Autodesk Inventor part; units mm, degrees
ref_plane "YZ Plane" through (0, 0, 0) normal (1, 0, 0) x (0, 1, 0)
ref_plane "XZ Plane" through (0, 0, 0) normal (0, 1, 0) x (-1, 0, 0)
ref_plane "XY Plane" through (0, 0, 0) normal (0, 0, 1) x (1, 0, 0)
sketch "Sketch1" plane through (0, 0, 0) normal (0, 1, 0) x (-1, 0, 0)
  line L0 (5, 5) -> (-5, 5)
  line L1 (-5, 5) -> (-5, -5)
  line L2 (-5, -5) -> (5, -5)
  line L3 (5, -5) -> (5, 5)
  point P0 (0, 0)
  dimension "d0" = 10
  dimension "d1" = 10
extrude "Extrusion1" add sketch "Sketch1" along normal blind 10
sketch "Sketch2" plane through (5, 0, 5) normal (1, 0, 0) x (0, 0, -1)
  line L0 (0, 0) -> (10, 0) construction
  line L1 (10, 0) -> (10, 10) construction
  line L2 (0, 10) -> (10, 10) construction
  line L3 (0, 0) -> (0, 10) construction
  line L4 (0, 10) -> (10, 10) construction
  line L5 (5, 10) -> (5, 0) construction
  line L6 (0, 0) -> (0, 10) construction
  line L7 (0, 5) -> (10, 5) construction
  line L8 (10, 0) -> (10, 10) construction
  circle A0 centre (5, 5) radius 2.5
  dimension "d4" = 5
extrude "Extrusion2" cut sketch "Sketch2" against normal blind 2
properties part number "cubo_calibracion_1cm"
Geometry check sheet. Reference: the model listing, model coordinates, mm. A direction names the side the tool comes from. Give positions to 0.01 mm unless a question says otherwise; leave off trailing zeros. Write each loop counter-clockwise with the first axis right and the second up, starting at its lowest first coordinate (ties: lowest second). Pieces come first, ordered by that corner, then holes. Notation, with made-up numbers: M -39.75,-30.5 L 8.25,-30.5 A22 ccw 8.25,-18.5 Z; hole C -10.5,70.25 d3. An arc over 180 degrees is marked long. One line per question, with ' | ' between items.
1. Cross-section at A-A (y = 6.5). Enter the section's corners in (x, z).
Ans:
outline: M -5,-5 L 5,-5 L 5,-2 L 3,-2 L 3,2 L 5,2 L 5,5 L -5,5 Z
2. Gauge pin test, flat end, axial feed: pin 1 (1.5 mm diameter, centred on y = 5.5, z = 1, fed in from +X). Record the tip position at first contact, or that the pin passes through.
Ans:
pin 1: x = 3
3. Cross-section at B-B (z = 0). Enter the section's corners in (x, y).
Ans:
outline: M -5,0 L 5,0 L 5,2.5 L 3,2.5 L 3,7.5 L 5,7.5 L 5,10 L -5,10 Z
4. Set-up check for faces 4 (the face through (4.01, 7.48, 0.33)), 5 (the face through (0, 0, 0)): record each of +Z, -Z, +X, -X, +Y, -Y from which the full face is reachable in a straight line by a thin tool's end or side.
Ans:
face 4: +X | face 5: +Z, -Z, +X, -X, -Y
5. Mould release check, pull along Y, two halves, no side actions. Record for faces 1 (the face through (0, 10, 0)), 2 (the face through (-5, 5, 0)), 3 (the face through (3, 5, 0)): released by +Y, released by -Y, zero draft, split by the parting line, or undercut.
Ans:
face 1: released by +Y | face 2: zero draft | face 3: undercut
6. Scan lines: line 1 along Y through (x, z) = (3.55, 0); line 2 along X through (y, z) = (5.25, -1.75); line 3 along Z through (x, y) = (4, 5.25). Record each from-to range of solid material in increasing order. Write a range as from..to.
Ans:
line 1: 0..2.5, 7.5..10 | line 2: -5..3 | line 3: -5..-2.49, 2.49..5
